For this review, take the finished solid that the model builds, in its own axes (mm). A direction names the side the tool comes from. Coordinates: 2 decimals unless noted, no trailing zeros. Write each loop counter-clockwise with the first axis right and the second up, starting at its lowest first coordinate (ties: lowest second). Pieces come first, ordered by that corner, then holes. Notation, with made-up numbers: M 23,-11 L 33,-11 A15 ccw 33,17 Z; hole C 88.25,56 d11. An arc over 180 degrees is marked long. Return JSON: item names as keys, results as strings.
```python
from build123d import *

# Parameters (mm, degrees)
SKETCH1_W                = 18
SKETCH1_H                = 40
BOSS_EXTRUDE1_DEPTH      = 5
BOSS_EXTRUDE2_DEPTH      = 14
SKETCH3_R                = 4.125
CUT_EXTRUDE1_DEPTH       = 30.017236257
FILLET1_R                = 7
SKETCH6_R                = 2.625
CUT_EXTRUDE3_DEPTH       = 33.939338184
SKETCH7_W                = 15.875
SKETCH7_H                = 5
BOSS_EXTRUDE3_DEPTH      = 7
FILLET2_R                = 7
SKETCH8_R                = 2.625
CUT_EXTRUDE4_DEPTH       = 30.189039039
BOSS_EXTRUDE4_DEPTH      = 2.5
BOSS_EXTRUDE4_DEPTH_BACK = 2.5


with BuildPart() as part:
    # Sketch1 → Boss-Extrude1 (new body)
    with BuildSketch(Plane(origin=(0, 0, 0), x_dir=(1, 0, 0), z_dir=(0, 1, 0))):
        Rectangle(SKETCH1_W, SKETCH1_H)
    extrude(amount=BOSS_EXTRUDE1_DEPTH)

    # Sketch2 → Boss-Extrude2 (add)
    with BuildSketch(Plane(origin=(0, 5, 0), x_dir=(1, 0, 0), z_dir=(0, 1, 0))):
        with BuildLine():
            Line((4, -20), (4, -8.660254038))
            ThreePointArc((4, -8.660254038), (-1, 0), (4, 8.660254038))
            Line((4, 8.660254038), (4, 20))
            Line((4, 20), (9, 20))
            Line((9, 20), (9, -20))
            Line((9, -20), (4, -20))
        make_face()
    extrude(amount=BOSS_EXTRUDE2_DEPTH)

    # Sketch3 → Cut-Extrude1 (cut, through all)
    with BuildSketch(Plane(origin=(0, 19, 0), x_dir=(1, 0, 0), z_dir=(0, 1, 0))):
        with Locations((9, 0)):
            Circle(SKETCH3_R)
    extrude(amount=-CUT_EXTRUDE1_DEPTH, mode=Mode.SUBTRACT)

    # Fillet1
    fillet1_edges = [part.edges().sort_by_distance(p)[0] for p in [
        (6.5, 19, 20),
        (6.5, 19, -20),
    ]]
    fillet(fillet1_edges, radius=FILLET1_R)

    # Sketch6 → Cut-Extrude3 (cut, through all)
    with BuildSketch(Plane(origin=(9, 0, 0), x_dir=(0, 0, -1), z_dir=(1, 0, 0))):
        with Locations((-13, 12)):
            Circle(SKETCH6_R)
        with Locations((13, 12)):
            Circle(SKETCH6_R)
    extrude(amount=-CUT_EXTRUDE3_DEPTH, mode=Mode.SUBTRACT)

    # Sketch7 → Boss-Extrude3 (add)
    with BuildSketch(Plane(origin=(9, 0, 0), x_dir=(0, 0, -1), z_dir=(1, 0, 0))):
        with Locations((-12.0625, 2.5)):
            Rectangle(SKETCH7_W, SKETCH7_H)
        with Locations((12.0625, 2.5)):
            Rectangle(SKETCH7_W, SKETCH7_H)
    extrude(amount=BOSS_EXTRUDE3_DEPTH)

    # Fillet2
    fillet2_edges = [part.edges().sort_by_distance(p)[0] for p in [
        (-9, 2.5, -20),
        (16, 2.5, -20),
        (16, 2.5, 20),
        (-9, 2.5, 20),
        (16, 2.5, -4.125),
        (16, 2.5, 4.125),
    ]]
    fillet(fillet2_edges, radius=FILLET2_R - 0.0001)  # a hair under: the kernel refuses the full size

    # Sketch8 → Cut-Extrude4 (cut, through all)
    with BuildSketch(Plane(origin=(0, 5, 0), x_dir=(1, 0, 0), z_dir=(0, 1, 0))):
        with Locations(Location((-2, 13, 0), (0, 0, 270))):
            Circle(SKETCH8_R)
        with Locations(Location((-2, -13, 0), (0, 0, 90))):
            Circle(SKETCH8_R)
    extrude(amount=-CUT_EXTRUDE4_DEPTH, mode=Mode.SUBTRACT)

    # Sketch9 → Boss-Extrude4 (add, two sides: drawn at the far end of the back side and taken through both)
    with BuildSketch(Plane.XY.offset(-BOSS_EXTRUDE4_DEPTH_BACK)):
        Polygon((-9, 5), (2, 16), (2, 5), align=None)
    extrude(amount=BOSS_EXTRUDE4_DEPTH + BOSS_EXTRUDE4_DEPTH_BACK)


solid = part.part
```
1. We need section D-D (z = 3). State the section outline as (x, y) points, plus the area to 3 significant figures.
Checks:
{"outline": "M -9,0 L 6.17,0 L 6.17,19 L -0.54,19 L -0.54,5 L -9,5 Z", "area": "170 mm2"}
2. Clearance check with flat-ended pins moving along their axes: pin 1 Ø3.5 at (x, z) = (12, -12.5) entering from +Y; pin 2 Ø6 at (y, z) = (9.5, -11) entering from +X; pin 3 Ø9 at (y, z) = (10.5, 15.5) entering from -X. State where each tip first meets the part, or that it passes through.
Checks:
{"pin 1": "y = 5", "pin 2": "x = 9", "pin 3": "x = 4"}
3. We need section B-B (y = 6.5). State the section outline as (x, z) points (3 decimals).
Checks:
{"outline": "M -7.5,-2.5 L -0.682,-2.5 A10 ccw 4,-8.66 L 4,-20 L 9,-20 L 9,-4.125 A4.125 cw 9,4.125 L 9,20 L 4,20 L 4,8.66 A10 ccw -0.682,2.5 L -7.5,2.5 Z"}
4. Draft analysis for pull direction Z (two halves, no side actions). For faces 1 (the face through (4, 12, 16)), 2 (the face through (-2.115, 2.535, 15.622)), 3 (the face through (14.004, 2.535, -6.23)), 4 (the face through (-3, 7, -2.5)), state which applies: +Z half, -Z half, draft (parallel to the pull), parting line (faces both ways), or undercut.
Checks:
{"face 1": "draft", "face 2": "undercut", "face 3": "undercut", "face 4": "-Z half"}
5. We need section A-A (x = 3). State the section outline as (y, z) points.
Checks:
{"outline": "M 0,-20 L 5,-20 L 5,-8 L 19,-8 L 19,8 L 5,8 L 5,20 L 0,20 Z"}
6. Wall thickness on L1, parallel to X at y = 2.05, z = 13 (3 decimals); L2, parallel to Y at x = 7.2, z = 13 (3 decimals); L3, parallel to X at y = 9.25, z = 15: over which ranges is each line inside the solid? List them lowest first. Write a range as from..to.
Checks:
{"L1": "-9..-4.625, 0.625..16", "L2": "0..9.375, 14.625..19", "L3": "4..9"}
7. We need section C-C (y = 2). Give the number of separate pieces and of enclosed holes in the cut face, plus the area to 3 significant figures.
Checks:
{"separate pieces": "1", "enclosed holes": "2", "area": "809 mm2"}
8. For faces 5 (the face through (16, 3, -12)), 6 (the face through (12, 5, -12)), 7 (the face through (-4, 5, 11)), 8 (the face through (-1, 13.5, 0.1)), 9 (the face through (4, 10, -16)), list the 3-axis set-ups (+Z, -Z, +X, -X, +Y, -Y) from which the entire face can be reached by the end or side of a thin tool; tool diameter is ignored.
Checks:
{"face 5": "+Z, -Z, +X, +Y, -Y", "face 6": "+Z, -Z, +X, +Y", "face 7": "+Z, -X, +Y", "face 8": "-X, +Y", "face 9": "-Z, -X, +Y"}
